Read the model definition and answer for the solid it produces. Units are mm, in the model's axes. Give positions to 0.01 mm unless a question says otherwise; leave off trailing zeros. Write each loop counter-clockwise with the first axis right and the second up, starting at its lowest first coordinate (ties: lowest second). Pieces come first, ordered by that corner, then holes. Notation, with made-up numbers: (0, -32) -> (5, -32) arc R21 cw to (5, -28) -> close; hole circle Ø3 at (87, -15.5). An arc over 180 degrees is marked (long way). Write item = value, one per line.
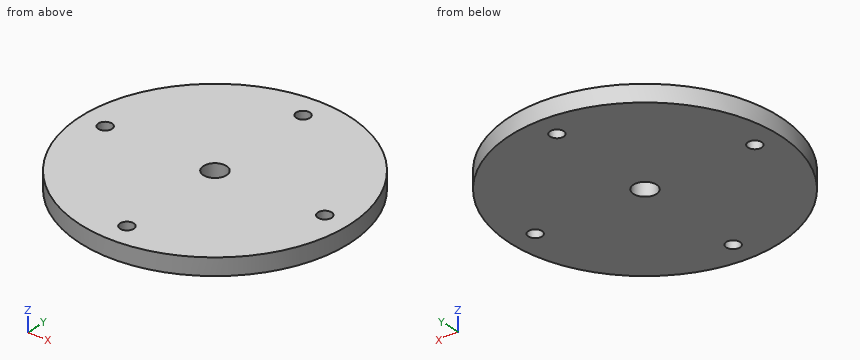
from build123d import *

# Parameters (mm, degrees)
SKETCH1_R           = 34.925
SKETCH1_R_2         = 3
SKETCH1_R_3         = 1.778
BOSS_EXTRUDE1_DEPTH = 4.3942


with BuildPart() as part:
    # Sketch1 → Boss-Extrude1 (new body)
    with BuildSketch(Plane.XY):
        Circle(SKETCH1_R)
        Circle(SKETCH1_R_2, mode=Mode.SUBTRACT)
        with Locations((0, 28.575)):
            Circle(SKETCH1_R_3, mode=Mode.SUBTRACT)
        with Locations((28.575, 0)):
            Circle(SKETCH1_R_3, mode=Mode.SUBTRACT)
        with Locations((0, -28.575)):
            Circle(SKETCH1_R_3, mode=Mode.SUBTRACT)
        with Locations((-28.575, 0)):
            Circle(SKETCH1_R_3, mode=Mode.SUBTRACT)
    extrude(amount=BOSS_EXTRUDE1_DEPTH)


solid = part.part
(1) The part is cut by section A-A on y = 0. Determine the outline of the cut face in (x, z) (3 decimals).
Checks:
outline = (-34.925, 0) -> (-30.353, 0) -> (-30.353, 4.394) -> (-34.925, 4.394) -> close; (-26.797, 0) -> (-3, 0) -> (-3, 4.394) -> (-26.797, 4.394) -> close; (3, 0) -> (26.797, 0) -> (26.797, 4.394) -> (3, 4.394) -> close; (30.353, 0) -> (34.925, 0) -> (34.925, 4.394) -> (30.353, 4.394) -> close
(2) The part is cut by section D-D on y = -15. Determine the outline of the cut face in (x, z).
Checks:
outline = (-31.54, 0) -> (31.54, 0) -> (31.54, 4.39) -> (-31.54, 4.39) -> close
(3) Given P1, Ø1.5, axis at y = 17.5, z = 3, coming from the -X side; P2, Ø2, axis at x = 23, z = 1.5, coming from the -Y side; P3, Ø12, axis at x = 22, y = -22.5, coming from the -Z side, each flat-ended and moving along its own axis, determine where each tip first touches the part or whether it passes through.
Checks:
P1 = -30.65
P2 = -27.12
P3 = 0
(4) The part is cut by section C-C on z = 3.25. Determine the outline of the cut face in (x, y) (3 decimals), plus the area to 3 significant figures.
Checks:
outline = circle Ø69.85 at (0, 0); hole circle Ø3.556 at (-28.575, 0); hole circle Ø6 at (0, 0); hole circle Ø3.556 at (0, -28.575); hole circle Ø3.556 at (0, 28.575); hole circle Ø3.556 at (28.575, 0)
area = 3,760 mm²
(5) Consider L1, parallel to Y at x = 0, z = 2.6 (3 decimals); L2, parallel to Y at x = -14, z = 1.85; L3, parallel to X at y = 6, z = 2.2. Determine where each line is inside the solid, lowest interval first.
Checks:
L1 = -34.925 to -30.353, -26.797 to -3, 3 to 26.797, 30.353 to 34.925
L2 = -32 to 32
L3 = -34.41 to 34.41
